```python
from build123d import *

# Parameters (mm, degrees)
F0_R          = 10
F1_DEPTH      = 100
F2_R          = 10
F3_DEPTH      = 20
F3_TAPER      = 15
F5_R          = 5
F6_DEPTH      = 80
F6_DEPTH_BACK = 3
F8_R          = 5
F9_DEPTH      = 80
F9_DEPTH_BACK = 3
F10_SIZE      = 0.5


with BuildPart() as f1:
    # F0 (on Front) → F1 (new body)
    with BuildSketch(Plane.XZ):
        Circle(F0_R)
    extrude(amount=F1_DEPTH)

    # F2 (on face) → F3 (join)
    with BuildSketch(Plane.XZ.offset(100)):
        Circle(F2_R)
    extrude(amount=F3_DEPTH, taper=F3_TAPER)

    # F5 (on offset) → F6 (join, two sides)
    with BuildSketch(Plane.YZ.offset(10)) as f6_sk:
        with Locations((-15, 0)):
            Circle(F5_R)
    extrude(amount=F6_DEPTH)
    extrude(f6_sk.sketch, amount=-F6_DEPTH_BACK)

    # F8 (on offset) → F9 (join, two sides)
    with BuildSketch(Plane.YZ.offset(-10)) as f9_sk:
        with Locations((-15, 0)):
            Circle(F8_R)
    extrude(amount=-F9_DEPTH)
    extrude(f9_sk.sketch, amount=F9_DEPTH_BACK)

    # F10
    f10_edges = [f1.edges().sort_by_distance(p)[0] for p in [
        (-90, -20, 0),
        (-10, 0, 0),
        (90, -20, 0),
    ]]
    chamfer(f10_edges, length=F10_SIZE)


solid = f1.part
```
Here's how the part is built. I have some questions about the finished solid (model axes, mm). A direction names the side the tool comes from. Round coordinates to 2 decimals unless told otherwise and drop trailing zeros. Order: outer loops, then holes, each group sorted by start corner. A loop starts at its lowest first (then second) coordinate and runs counter-clockwise, first axis right, second up. Notation, with made-up numbers: (53.5, -6) -> (65.5, -6) arc R28 cw to (65.5, 25) -> close; hole circle Ø1 at (11.5, -2). An arc over 180 degrees is marked (long way). Use a Markdown table: item, result. Add a question column.
(1) Suppose I cut it at C-C, the plane y = -34.5. Please give me the cut outline in (x, z).
(2) Suppose I cut it at A-A, the plane y = -15. Please give me the cut outline in (x, z).
(3) For faces 1 (the face through (90, -15, 0)), 2 (the face through (-50, -20, 0)), which set-ups out of +Z, -Z, +X, -X, +Y, -Y let a thin tool reach every point of the face, with its end or its side?
(4) I need wall thicknesses on line 1 along Y through (x, z) = (-42.5, -0.5); line 2 along Y through (x, z) = (55, 1); line 3 along Z through (x, y) = (6.5, -104.5). Which ranges of each line are inside material? Lowest first, please.
(5) For pin 1 Ø5 at (x, z) = (-25.5, -1.5) entering from -Y; pin 2 Ø3 at (x, z) = (41.5, 4.5) entering from +Y; pin 3 Ø3 at (x, z) = (-30, 4.5) entering from -Y, each with a flat end and sliding along its axis, tell me the tip position at first contact or that it passes through.
(6) Suppose I cut it at B-B, the plane x = 0. Please give me the cut outline in (y, z).
(7) Suppose I cut it at D-D, the plane x = 58. Please give me the cut outline in (y, z).
Verdict:
| question | item | result |
|---|---|---|
| 1 | outline | circle Ø20 at (0, 0) |
| 2 | outline | (-90, -4.5) -> (-89.5, -5) -> (-8.66, -5) arc R10 ccw to (8.66, -5) -> (89.5, -5) -> (90, -4.5) -> (90, 4.5) -> (89.5, 5) -> (8.66, 5) arc R10 ccw to (-8.66, 5) -> (-89.5, 5) -> (-90, 4.5) -> close |
| 3 | face 1 | +Z, -Z, +X, +Y, -Y |
| 3 | face 2 | -X |
| 4 | line 1 | -19.97 to -10.03 |
| 4 | line 2 | -19.9 to -10.1 |
| 4 | line 3 | -5.92 to 5.92 |
| 5 | pin 1 | y = -20 |
| 5 | pin 2 | y = -11 |
| 5 | pin 3 | y = -19 |
| 6 | outline | (-120, -4.64) -> (-100, -10) -> (-0.5, -10) -> (0, -9.5) -> (0, 9.5) -> (-0.5, 10) -> (-100, 10) -> (-120, 4.64) -> close |
| 7 | outline | circle Ø10 at (-15, 0) |
